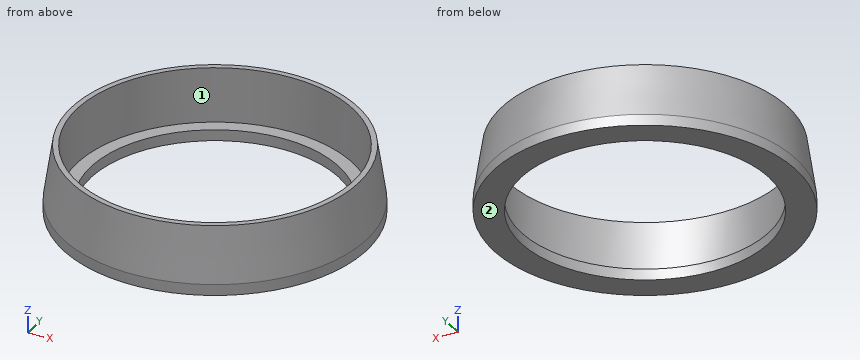
```python
from build123d import *

# Parameters (mm, degrees)
SKETCH_1_R      = 27.5
SKETCH_1_R_2    = 22.5
EXTRUDE_1_DEPTH = 2


with BuildPart() as part:
    # 草圖5 → 旋轉2 (revolve)
    with BuildSketch(Plane(origin=(0, 0, 0), x_dir=(0, 0, -1), z_dir=(1, 0, 0))):
        Polygon((-10, 26), (0, 27.5), (0, 25), (-10, 25), align=None)
    revolve(axis=Axis((0, 0, 10), (0, 0, -1)))

    # 草圖1 → 填料-伸長1 (add)
    with BuildSketch(Plane.XY):
        Circle(SKETCH_1_R)
        Circle(SKETCH_1_R_2, mode=Mode.SUBTRACT)
    extrude(amount=-EXTRUDE_1_DEPTH)


solid = part.part
```
Part model, mm, in its own coordinate system. Face numbers are marked on the shaded views. A direction names the side the tool comes from. Round coordinates to 2 decimals unless told otherwise and drop trailing zeros. Write each loop counter-clockwise with the first axis right and the second up, starting at its lowest first coordinate (ties: lowest second). Pieces come first, ordered by that corner, then holes.
Item 1: Drop flat-ended pins along their axis: pin 1 Ø25 at (x, y) = (-6.5, 7.5) entering from +Z; pin 2 Ø5 at (y, z) = (4.5, 4.5) entering from -X; pin 3 Ø4 at (y, z) = (18, 5) entering from +X; pin 4 Ø10 at (x, y) = (-10.5, 16.5) entering from +Z. Give the stop position or say it passes through.
Results:
pin 1: passes through
pin 2: stops at x = -26.96
pin 3: stops at x = 21.48
pin 4: stops at z = 0
Item 2: Cut at C-C, the plane z = 2. Give the cut face in (x, y).
Results:
outline: circle Ø54.4 at (0, 0); hole circle Ø50 at (0, 0)
Item 3: Probe L1, parallel to Y at x = 0, z = -0.95; L2, parallel to Z at x = 7.5, y = -23; L3, parallel to X at y = 19.5, z = -0.25. List the from-to ranges inside material, lowest first.
Results:
L1: y = -27.5 to -22.5, 22.5 to 27.5
L2: z = -2 to 0
L3: x = -19.39 to -11.22, 11.22 to 19.39
Item 4: Cut at A-A, the plane y = 0. Give the cut face in (x, z).
Results:
outline: (-27.5, -2) - (-22.5, -2) - (-22.5, 0) - (-25, 0) - (-25, 10) - (-26, 10) - (-27.5, 0) - close; (22.5, -2) - (27.5, -2) - (27.5, 0) - (26, 10) - (25, 10) - (25, 0) - (22.5, 0) - close
Item 5: Which spindle directions (+Z, -Z, +X, -X, +Y, -Y) get a long thin tool onto all of the face, cutting with end or side? Do the marked faces 1 and 2. Say none if no direction does.
Results:
face 1: +Z
face 2: -Z, +X, -X, +Y, -Y
